Could you check a few things on this model? Use its own coordinates, in mm. Face numbers are marked on the shaded views. Give positions to 0.01 mm unless a question says otherwise; leave off trailing zeros. Loops run counter-clockwise (first coordinate to the right, second up) from the corner with the lowest first, then second, coordinate; pieces in that order, holes last.
1. Imagine slicing it at B-B (y = 174). List the corners of the cut face in (x, z) for me.
2. Imagine slicing it at D-D (z = -621). List the corners of the cut face in (x, y) for me.
3. Thinking about a two-plate mould opening in X: for the marked faces 1 and 2, which applies, +X half, -X half, draft (parallel to the pull), parting line (faces both ways), or undercut?
4. For P1, Ø5, axis at y = 605.5, z = -96, coming from the +X side; P2, Ø5, axis at y = 115.5, z = -444, coming from the -X side; P3, Ø11, axis at x = 1646, y = 603, coming from the +Z side, each with a flat end and sliding along its axis, tell me the tip position at first contact or that it passes through.
5. I need wall thicknesses on line 1 along X through (y, z) = (430, -99); line 2 along Y through (x, z) = (1047, -65); line 3 along X through (y, z) = (565, -250). Which ranges of each line are inside material? Lowest first, please.
6. Imagine slicing it at C-C (x = 1583.5). List the corners of the cut face in (y, z) for me, plus the area to 3 significant figures.
7. Imagine slicing it at A-A (z = -475). List the corners of the cut face in (x, y) for me, plus the area to 3 significant figures.
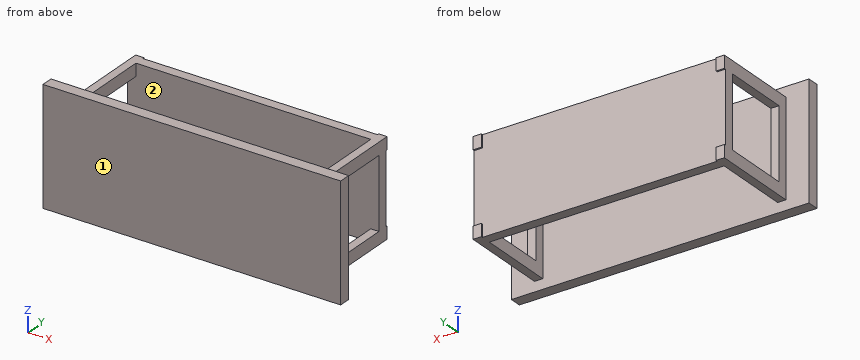
```python
from build123d import *

# Parameters (mm, degrees)
SKETCH_1_W      = 1800
SKETCH_1_H      = 700
EXTRUDE_1_DEPTH = 70
SKETCH_2_W      = 50
SKETCH_2_H      = 580
EXTRUDE_2_DEPTH = 60
SKETCH_3_W      = 50
SKETCH_3_H      = 75
EXTRUDE_3_DEPTH = 480
EXTRUDE_4_REACH = 1984.757
SKETCH_4_W      = 50
SKETCH_4_H      = 60
EXTRUDE_5_REACH = 1860.548
SKETCH_5_W      = 580
SKETCH_5_H      = 60


with BuildPart() as part:
    # ｽｹｯﾁ1 → ﾎﾞｽ - 押し出し1 (new body)
    with BuildSketch(Plane(origin=(0, 0, 0), x_dir=(1, 0, 0), z_dir=(0, 1, 0))):
        with Locations((900, 350)):
            Rectangle(SKETCH_1_W, SKETCH_1_H)
    extrude(amount=EXTRUDE_1_DEPTH)

    # ｽｹｯﾁ2 → ﾎﾞｽ - 押し出し2 (add)
    with BuildSketch(Plane(origin=(0, 70, 0), x_dir=(1, 0, 0), z_dir=(0, 1, 0))):
        with Locations((165, 350)):
            Rectangle(SKETCH_2_W, SKETCH_2_H)
        with Locations((1635, 350)):
            Rectangle(SKETCH_2_W, SKETCH_2_H)
    extrude(amount=EXTRUDE_2_DEPTH)

    # ｽｹｯﾁ3 → ﾎﾞｽ - 押し出し3 (add)
    with BuildSketch(Plane(origin=(0, 130, 0), x_dir=(1, 0, 0), z_dir=(0, 1, 0))):
        with Locations((165, 602.5)):
            Rectangle(SKETCH_3_W, SKETCH_3_H)
        with Locations((165, 97.5)):
            Rectangle(SKETCH_3_W, SKETCH_3_H)
        with Locations((1635, 602.5)):
            Rectangle(SKETCH_3_W, SKETCH_3_H)
        with Locations((1635, 97.5)):
            Rectangle(SKETCH_3_W, SKETCH_3_H)
    extrude(amount=EXTRUDE_3_DEPTH)

    # ｽｹｯﾁ4 → ﾎﾞｽ - 押し出し4 (add, up to next)
    with BuildSketch(Plane.XY.offset(-565), mode=Mode.PRIVATE) as extrude_4_sk1:
        with Locations((1635, 570)):
            Rectangle(SKETCH_4_W, SKETCH_4_H)
    extrude_4_tool1 = extrude(extrude_4_sk1.sketch, amount=EXTRUDE_4_REACH, mode=Mode.PRIVATE) - part.part
    # ｽｹｯﾁ4 → ﾎﾞｽ - 押し出し4 (add, up to next)
    with BuildSketch(Plane.XY.offset(-565), mode=Mode.PRIVATE) as extrude_4_sk2:
        with Locations((165, 570)):
            Rectangle(SKETCH_4_W, SKETCH_4_H)
    extrude_4_tool2 = extrude(extrude_4_sk2.sketch, amount=EXTRUDE_4_REACH, mode=Mode.PRIVATE) - part.part
    add(extrude_4_tool1.solids().sort_by_distance((1635, 570, -565))[0])
    add(extrude_4_tool2.solids().sort_by_distance((165, 570, -565))[0])

    # ｽｹｯﾁ5 → ﾎﾞｽ - 押し出し5 (add, up to next)
    with BuildSketch(Plane.ZY.offset(-1610), mode=Mode.PRIVATE) as extrude_5_sk1:
        with Locations((-350, 570)):
            Rectangle(SKETCH_5_W, SKETCH_5_H)
    extrude_5_tool1 = extrude(extrude_5_sk1.sketch, amount=EXTRUDE_5_REACH, mode=Mode.PRIVATE) - part.part
    add(extrude_5_tool1.solids().sort_by_distance((1610, 570, -350))[0])


solid = part.part
```
Derived:
1. outline: (140, -640) - (190, -640) - (190, -565) - (140, -565) - close; (140, -135) - (190, -135) - (190, -60) - (140, -60) - close; (1610, -640) - (1660, -640) - (1660, -565) - (1610, -565) - close; (1610, -135) - (1660, -135) - (1660, -60) - (1610, -60) - close
2. outline: (0, 0) - (1800, 0) - (1800, 70) - (1660, 70) - (1660, 610) - (1610, 610) - (1610, 600) - (190, 600) - (190, 610) - (140, 610) - (140, 70) - (0, 70) - close; hole (190, 70) - (1610, 70) - (1610, 540) - (190, 540) - close
3. face 1: draft
3. face 2: undercut
4. P1: stops at x = 1660
4. P2: stops at x = 140
4. P3: stops at z = -60
5. line 1: x = 140 to 190, 1610 to 1660
5. line 2: y = 0 to 70, 540 to 600
5. line 3: x = 140 to 1660
6. outline: (0, -700) - (70, -700) - (70, 0) - (0, 0) - close; (540, -640) - (600, -640) - (600, -60) - (540, -60) - close
6. area: 83,800 mm2
7. outline: (0, 0) - (1800, 0) - (1800, 70) - (1660, 70) - (1660, 130) - (1610, 130) - (1610, 70) - (190, 70) - (190, 130) - (140, 130) - (140, 70) - (0, 70) - close; (140, 540) - (1660, 540) - (1660, 600) - (140, 600) - close
7. area: 223,000 mm2
